```python
from build123d import *

# Parameters (mm, degrees)
SKETCH1_R           = 3.5
BOSS_EXTRUDE1_DEPTH = 3.5
SKETCH2_W           = 15
SKETCH2_H           = 3.5
CUT_EXTRUDE1_DEPTH  = 45.343122353


with BuildPart() as part:
    # Sketch1 → Boss-Extrude1 (new body)
    with BuildSketch(Plane.XY):
        Polygon((27.25, -26), (27.25, -22.5), (32.25, -22.5), (32.25, -11), (35.75, -11), (35.75, -7.5), (32.25, -7.5), (32.25, 7.5), (35.75, 7.5), (35.75, 11), (32.25, 11), (32.25, 22.5), (27.25, 22.5), (27.25, 26), (12.25, 26), (12.25, 22.5), (-12.25, 22.5), (-12.25, 26), (-27.25, 26), (-27.25, 22.5), (-32.25, 22.5), (-32.25, -22.5), (-27.25, -22.5), (-27.25, -26), (-12.25, -26), (-12.25, -22.5), (12.25, -22.5), (12.25, -26), align=None)
        Circle(SKETCH1_R, mode=Mode.SUBTRACT)
        with BuildLine():
            Line((1, 19), (1, 7))
            ThreePointArc((1, 7), (0, 6), (-1, 7))
            Line((-1, 7), (-1, 19))
            ThreePointArc((-1, 19), (0, 20), (1, 19))
        make_face(mode=Mode.SUBTRACT)
        with BuildLine():
            Line((1, -19), (1, -7))
            ThreePointArc((1, -7), (0, -6), (-1, -7))
            Line((-1, -7), (-1, -19))
            ThreePointArc((-1, -19), (0, -20), (1, -19))
        make_face(mode=Mode.SUBTRACT)
    extrude(amount=BOSS_EXTRUDE1_DEPTH)

    # Sketch2 → Cut-Extrude1 (cut, through all)
    with BuildSketch(Plane(origin=(0, 0, 0), x_dir=(-1, 0, 0), z_dir=(0, 0, -1))):
        with Locations((19.65, -0.25)):
            Rectangle(SKETCH2_W, SKETCH2_H)
        with Locations((-19.75, -0.25)):
            Rectangle(SKETCH2_W, SKETCH2_H)
    extrude(amount=-CUT_EXTRUDE1_DEPTH, mode=Mode.SUBTRACT)


solid = part.part
```
For this review, take the finished solid that the model builds, in its own axes (mm). A direction names the side the tool comes from. Coordinates: 2 decimals unless noted, no trailing zeros. Write each loop counter-clockwise with the first axis right and the second up, starting at its lowest first coordinate (ties: lowest second). Pieces come first, ordered by that corner, then holes.
(1) Add section C-C on y = -18. Give the boundary of the cut face in (x, z), then the cut area to 3 significant figures.
(2) Add section B-B on x = -19. Give the boundary of the cut face in (y, z).
(3) The part is to be moulded in two halves that separate along Y. For faces 1 (the face through (1, 6, 3.5)), 2 (the face through (30, -22.5, 2)), 3 (the face through (20, -2, 2)), say which applies: +Y half, -Y half, draft (parallel to the pull), parting line (faces both ways), or undercut.
(4) Tool access review of faces 4 (the face through (12.25, -24, 2)), 5 (the face through (34, -11, 2)), 6 (the face through (32.25, 0, 2)), 7 (the face through (-27.25, 24, 2)): name each direction out of +Z, -Z, +X, -X, +Y, -Y from which nothing blocks a thin tool from reaching the whole face with its end or side.
(5) Add section A-A on y = 0. Give the boundary of the cut face in (x, z).
(6) Add section D-D on x = 0. Give the boundary of the cut face in (y, z).
(7) Wall thickness on probe 1 along Y at (x, z) = (0, 1.9); probe 2 along Y at (x, z) = (-18.5, 0.25); probe 3 along X at (y, z) = (15, 1.15): over which ranges is each line inside the solid? List them lowest first.
(8) For pin 1 Ø1.8 at (x, z) = (33.5, 1.5) entering from +Y; pin 2 Ø1.8 at (y, z) = (-1, 1.5) entering from +X; pin 3 Ø1.5 at (x, y) = (2.5, 7.5) entering from -Z; pin 4 Ø1 at (x, z) = (-5.5, 2) entering from -Y, all flat-tipped, find the tip position at first contact; note any pin that passes through.
Answer sheet:
1. outline: (-32.25, 0) - (-1, 0) - (-1, 3.5) - (-32.25, 3.5) - close; (1, 0) - (32.25, 0) - (32.25, 3.5) - (1, 3.5) - close
1. area: 219 mm2
2. outline: (-26, 0) - (-2, 0) - (-2, 3.5) - (-26, 3.5) - close; (1.5, 0) - (26, 0) - (26, 3.5) - (1.5, 3.5) - close
3. face 1: draft
3. face 2: -Y half
3. face 3: undercut
4. face 4: +Z, -Z, -Y
4. face 5: +Z, -Z, +X, -Y
4. face 6: +Z, -Z, +X
4. face 7: +Z, -Z, -X, +Y
5. outline: (-32.25, 0) - (-27.15, 0) - (-27.15, 3.5) - (-32.25, 3.5) - close; (-12.15, 0) - (-3.5, 0) - (-3.5, 3.5) - (-12.15, 3.5) - close; (3.5, 0) - (12.25, 0) - (12.25, 3.5) - (3.5, 3.5) - close; (27.25, 0) - (32.25, 0) - (32.25, 3.5) - (27.25, 3.5) - close
6. outline: (-22.5, 0) - (-20, 0) - (-20, 3.5) - (-22.5, 3.5) - close; (-6, 0) - (-3.5, 0) - (-3.5, 3.5) - (-6, 3.5) - close; (3.5, 0) - (6, 0) - (6, 3.5) - (3.5, 3.5) - close; (20, 0) - (22.5, 0) - (22.5, 3.5) - (20, 3.5) - close
7. probe 1: y = -22.5 to -20, -6 to -3.5, 3.5 to 6, 20 to 22.5
7. probe 2: y = -26 to -2, 1.5 to 26
7. probe 3: x = -32.25 to -1, 1 to 32.25
8. pin 1: stops at y = 11
8. pin 2: stops at x = 32.25
8. pin 3: stops at z = 0
8. pin 4: stops at y = -22.5
